Here's how the part is built. I have some questions about the finished solid (model axes, mm). A direction names the side the tool comes from. Give positions to 0.01 mm unless a question says otherwise; leave off trailing zeros. Order: outer loops, then holes, each group sorted by start corner. A loop starts at its lowest first (then second) coordinate and runs counter-clockwise, first axis right, second up. Notation, with made-up numbers: M 8,86.25 L 35,86.25 A29 cw 35,113.25 Z; hole C -31.5,28 d4. An arc over 180 degrees is marked long. Use CSV: the item, a comma, the result in double quotes. Start each with the question number.
```python
from build123d import *

# Parameters (mm, degrees)
PAD_DEPTH       = 3
CHAMFER_SIZE    = 0.5
CHAMFER001_SIZE = 1


with BuildPart() as part:
    # Sketch → Pad (new body)
    with BuildSketch(Plane.XY):
        Polygon((-5.921, -13.5), (5.921, -13.5), (5.921, -8.5), (20, -8.5), (20, 8.5), (5.921, 8.5), (5.921, 13.5), (1.5, 19.5), (1.5, 128.5), (-1.5, 128.5), (-1.5, 19.5), (-5.921, 13.5), (-5.921, 8.5), (-20, 8.5), (-20, -8.5), (-5.921, -8.5), align=None)
        Polygon((2.921, -10.5), (-2.921, -10.5), (-2.921, -5.5), (-17, -5.5), (-17, 5.5), (-2.921, 5.5), (-2.921, 10.5), (2.921, 10.5), (2.921, 5.5), (17, 5.5), (17, -5.5), (2.921, -5.5), align=None, mode=Mode.SUBTRACT)
    extrude(amount=PAD_DEPTH)

    # Chamfer
    chamfer_edges = [part.edges().sort_by_distance(p)[0] for p in [
        (-2.921, 5.5, 1.5),
        (2.921, 5.5, 1.5),
        (-2.921, -5.5, 1.5),
        (2.921, -5.5, 1.5),
    ]]
    chamfer(chamfer_edges, length=CHAMFER_SIZE)

    # Chamfer001
    chamfer001_edges = [part.edges().sort_by_distance(p)[0] for p in [
        (1.5, 128.5, 1.5),
        (-1.5, 128.5, 1.5),
    ]]
    chamfer(chamfer001_edges, length=CHAMFER001_SIZE)


solid = part.part
```
Q1. For P1, Ø1.5, axis at y = 49, z = 1, coming from the -X side; P2, Ø0.9, axis at x = 1, z = 1.5, coming from the +Y side; P3, Ø1.5, axis at y = 10.5, z = 1, coming from the -X side, each with a flat end and sliding along its axis, tell me the tip position at first contact or that it passes through.
Q2. We'd pull the mould along X, two halves only. Please class faces 5 (the face through (10, -5.5, 1)), 6 (the face through (20, 0, 1)), 7 (the face through (0, 42, 0)), 8 (the face through (-1.5, 74, 1)): pulls with the +X half, pulls with the -X half, needs draft (parallel to the pull), parting line crosses it, or undercut.
Q3. Imagine slicing it at B-B, the plane y = 0. Please give me the cut outline in (x, z).
Q4. For faces 1 (the face through (-5.921, -11, 1)), 2 (the face through (-2.921, 8, 1)), 3 (the face through (-13, 8.5, 1)), 4 (the face through (13, 8.5, 1)), which set-ups out of +Z, -Z, +X, -X, +Y, -Y let a thin tool reach every point of the face, with its end or its side?
Q5. Imagine slicing it at D-D, the plane y = 61. Please give me the cut outline in (x, z).
Q6. Imagine slicing it at C-C, the plane x = 11.5. Please give me the cut outline in (y, z), then the cut area to 3 significant figures.
Q7. I need wall thicknesses on line 1 (Y direction, x = 16, z = 1.75); line 2 (X direction, y = 6.5, z = 1.95); line 3 (X direction, y = 22, z = 2.25). Which ranges of each line are inside material? Lowest first, please. Write a range as [from, to].
Reply:
1,P1,"stops at x = -1.5"
1,P2,"stops at y = 128.45"
1,P3,"stops at x = -5.92"
2,face 5,"undercut"
2,face 6,"pulls with the +X half"
2,face 7,"needs draft"
2,face 8,"pulls with the -X half"
3,outline,"M -20,0 L -17,0 L -17,3 L -20,3 Z; M 17,0 L 20,0 L 20,3 L 17,3 Z"
4,face 1,"+Z, -Z, -X, -Y"
4,face 2,"+Z, -Z"
4,face 3,"+Z, -Z, -X, +Y"
4,face 4,"+Z, -Z, +X, +Y"
5,outline,"M -1.5,0 L 1.5,0 L 1.5,3 L -1.5,3 Z"
6,outline,"M -8.5,0 L -5.5,0 L -5.5,3 L -8.5,3 Z; M 5.5,0 L 8.5,0 L 8.5,3 L 5.5,3 Z"
6,area,"18.0 mm^2"
7,line 1,"y = [-8.5, -5.5], [5.5, 8.5]"
7,line 2,"x = [-20, -2.92], [2.92, 20]"
7,line 3,"x = [-1.5, 1.5]"
